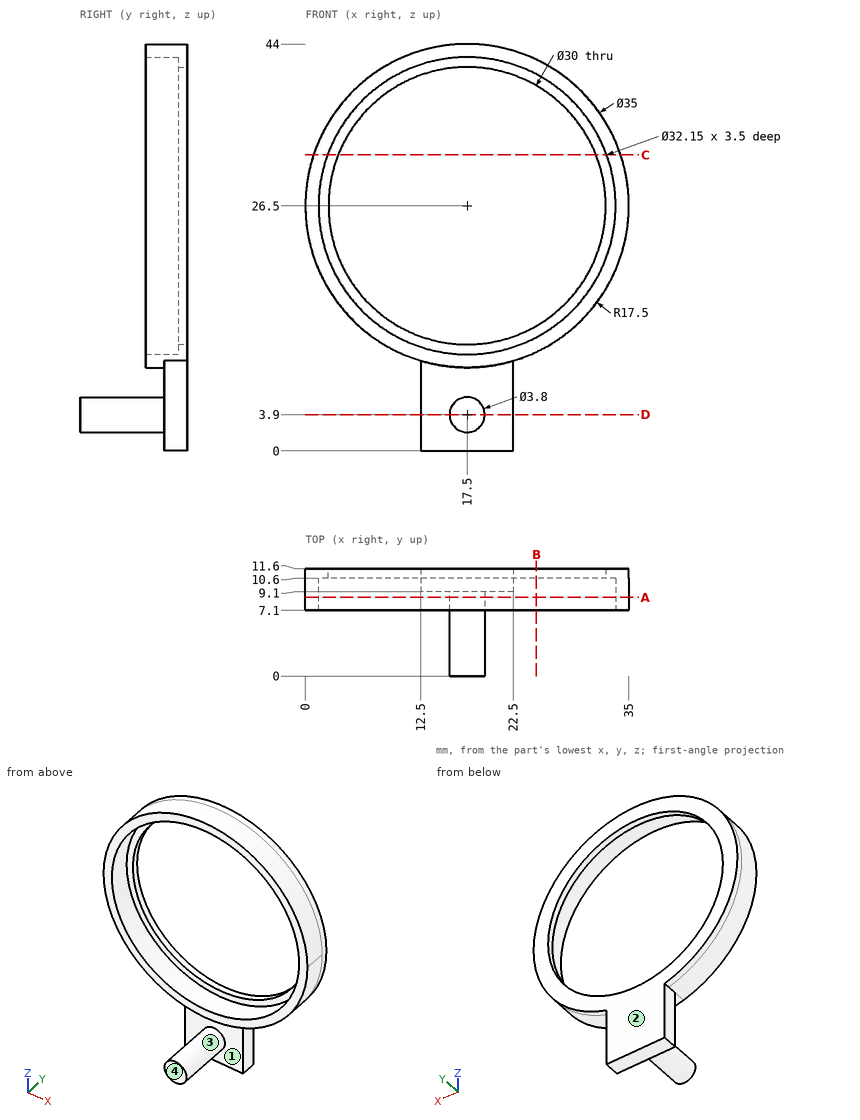
The figure shows three views and two pictorial views of one solid part (mm, origin at its lowest corner). Answer the questions. A direction names the side the tool comes from. Coordinates: 2 decimals unless noted, no trailing zeros. Loops run counter-clockwise (first coordinate to the right, second up) from the corner with the lowest first, then second, coordinate; pieces in that order, holes last.
1) Find section A-A on y = 8.5. Give the number of separate pieces and of enclosed holes in the cut face, then the cut area to 3 significant figures.
2) Find the intervals of material crossed by L1, parallel to Y at x = 19.5, z = 10; L2, parallel to Z at x = 17.5, y = 10.8; L3, parallel to Z at x = 30, y = 9, in increasing order.
3) Flat-ended cylindrical pins translate along their axes: pin 1 Ø5 at (x, y) = (12.5, 8) entering from +Z; pin 2 Ø3 at (y, z) = (7.5, 19.5) entering from +X; pin 3 Ø5 at (x, y) = (31.5, 9) entering from +Z. Find the tip coordinate at first contact, or state that the pin passes through.
4) Determine the mould class of the marked faces 1 and 2 for opening direction Z: pulls with the +Z half, pulls with the -Z half, needs draft (parallel to the pull), parting line crosses it, or undercut.
5) Find section C-C on z = 32. Write down the section's boundary in (x, y).
6) Find section D-D on z = 3.9. Write down the section's boundary in (x, y).
7) Find section B-B on x = 25. Write down the section's boundary in (y, z), then the cut area to 3 significant figures.
8) A tool of negligible diameter and unlimited length cuts with its end or side. For the marked faces 3 and 4, from which of +Z, -Z, +X, -X, +Y, -Y can it reach the whole face along a straight path? Write none if from no direction.
Values:
1. separate pieces: 2
1. enclosed holes: 1
1. area: 162 mm2
2. L1: y = 7.1 to 11.6
2. L2: z = 0 to 11.5, 41.5 to 44
2. L3: z = 14.25 to 16.39, 36.61 to 38.75
3. pin 1: stops at z = 43.82
3. pin 2: stops at x = 34.11
3. pin 3: stops at z = 39.69
4. face 1: undercut
4. face 2: needs draft
5. outline: (0.89, 7.1) - (2.4, 7.1) - (2.4, 10.6) - (3.54, 10.6) - (3.54, 11.6) - (0.89, 11.6) - close; (31.46, 10.6) - (32.6, 10.6) - (32.6, 7.1) - (34.11, 7.1) - (34.11, 11.6) - (31.46, 11.6) - close
6. outline: (12.5, 9.1) - (15.6, 9.1) - (15.6, 0) - (19.4, 0) - (19.4, 9.1) - (22.5, 9.1) - (22.5, 11.6) - (12.5, 11.6) - close
7. outline: (7.1, 10.69) - (11.6, 10.69) - (11.6, 13.51) - (10.6, 13.51) - (10.6, 12.28) - (7.1, 12.28) - close; (7.1, 40.72) - (10.6, 40.72) - (10.6, 39.49) - (11.6, 39.49) - (11.6, 42.31) - (7.1, 42.31) - close
7. area: 16.8 mm2
8. face 3: -Y
8. face 4: +Z, -Z, +X, -X, -Y
